Autodesk Fusion 360 part; units mm, degrees
sketch "Coupon chord" plane through (0, 0, 0) normal (0, 1, 0) x (1, 0, 0)
  line L0 (70, -76) -> (150, -76)
  line L1 (150, -76) -> (150, -90)
  line L2 (150, -90) -> (70, -90)
  line L3 (70, -90) -> (70, -76)
  dimension "d52" = 70
  dimension "d53" = 76
  dimension "d55" = 90
extrude "Coupon chord (1)" add sketch "Coupon chord" along normal mid plane 8
sketch "Saddle boss x=70" plane through (0, 0, 0) normal (0, 1, 0) x (1, 0, 0)
  circle A0 centre (70, -90) radius 22.7
  dimension "d58" = 70
  dimension "d59" = 90
  dimension "d60" = 45.4
extrude "Saddle boss x=70 (1)" add sketch "Saddle boss x=70" along normal mid plane 8
sketch "Saddle boss x=150" plane through (0, 0, 0) normal (0, 1, 0) x (1, 0, 0)
  circle A0 centre (150, -90) radius 22.7
  dimension "d64" = 90
  dimension "d65" = 45.4
extrude "Saddle boss x=150 (1)" add sketch "Saddle boss x=150" along normal mid plane 8
sketch "Rod pocket x=70" plane through (0, 0, 0) normal (0, 1, 0) x (1, 0, 0)
  circle A0 centre (70, -90) radius 17.1
  dimension "d68" = 70
  dimension "d69" = 90
  dimension "d70" = 34.2
extrude "Rod pocket x=70 (1)" cut sketch "Rod pocket x=70" along normal mid plane 18
sketch "Drop-in opening x=70" plane through (0, 0, 0) normal (0, 1, 0) x (1, 0, 0)
  line L0 (52.9, -90) -> (87.1, -90)
  line L1 (87.1, -90) -> (87.1, -117.7)
  line L2 (87.1, -117.7) -> (52.9, -117.7)
  line L3 (52.9, -117.7) -> (52.9, -90)
  dimension "d73" = 52.9
  dimension "d74" = 90
  dimension "d75" = 87.1
  dimension "d76" = 117.7
extrude "Drop-in opening x=70 (1)" cut sketch "Drop-in opening x=70" along normal mid plane 18
sketch "Rod pocket x=150" plane through (0, 0, 0) normal (0, 1, 0) x (1, 0, 0)
  circle A0 centre (150, -90) radius 17.1
  dimension "d80" = 90
  dimension "d81" = 34.2
extrude "Rod pocket x=150 (1)" cut sketch "Rod pocket x=150" along normal mid plane 18
sketch "Drop-in opening x=150" plane through (0, 0, 0) normal (0, 1, 0) x (1, 0, 0)
  line L0 (132.9, -90) -> (167.1, -90)
  line L1 (167.1, -90) -> (167.1, -117.7)
  line L2 (167.1, -117.7) -> (132.9, -117.7)
  line L3 (132.9, -117.7) -> (132.9, -90)
  dimension "d84" = 132.9
  dimension "d85" = 90
  dimension "d86" = 167.1
  dimension "d87" = 117.7
extrude "Drop-in opening x=150 (1)" cut sketch "Drop-in opening x=150" along normal mid plane 18
equation "couponWidth = 8.0 mm"
equation "plateHeight = 90.0 mm"
equation "rodOuterDiameter = 33.4 mm"
equation "saddleClearance = 0.8 mm"
equation "saddleWall = 6.0 mm"
equation "rearRodStandoff = 70.0 mm"
equation "rodSpacing = 80.0 mm"
equation "memberWidth = 14.0 mm"
equation "d52 = rearRodStandoff"
equation "d53 = plateHeight - memberWidth"
equation "d55 = plateHeight"
equation "d56 = couponWidth"
equation "d58 = rearRodStandoff"
equation "d59 = plateHeight"
equation "d60 = rodOuterDiameter + 2 * saddleWall"
equation "d61 = couponWidth"
equation "d64 = plateHeight"
equation "d65 = rodOuterDiameter + 2 * saddleWall"
equation "d66 = couponWidth"
equation "d68 = rearRodStandoff"
equation "d69 = plateHeight"
equation "d70 = rodOuterDiameter + saddleClearance"
equation "d71 = couponWidth + 10 mm"
equation "d73 = rearRodStandoff - ( rodOuterDiameter + saddleClearance ) / 2"
equation "d74 = plateHeight"
equation "d75 = rearRodStandoff + ( rodOuterDiameter + saddleClearance ) / 2"
equation "d76 = plateHeight + ( rodOuterDiameter + 2 * saddleWall ) / 2 + 5 mm"
equation "d77 = couponWidth + 10 mm"
equation "d80 = plateHeight"
equation "d81 = rodOuterDiameter + saddleClearance"
equation "d82 = couponWidth + 10 mm"
equation "d84 = ( rearRodStandoff + rodSpacing ) - ( rodOuterDiameter + saddleClearance ) / 2"
equation "d85 = plateHeight"
equation "d86 = ( rearRodStandoff + rodSpacing ) + ( rodOuterDiameter + saddleClearance ) / 2"
equation "d87 = plateHeight + ( rodOuterDiameter + 2 * saddleWall ) / 2 + 5 mm"
equation "d88 = couponWidth + 10 mm"
Model file for the job. Use its own axes, mm. A direction names the side the tool comes from. Give positions to 0.01 mm unless a question says otherwise; leave off trailing zeros. Loops run counter-clockwise (first coordinate to the right, second up) from the corner with the lowest first, then second, coordinate; pieces in that order, holes last.
1) Tool access for faces 4 (the flat face through (110, 0, 76)), 5 (the flat face through (132.9, 0, 98)), 6 (the cylindrical face through (164.86, 0.06, 72.84)): list every direction of +Z, -Z, +X, -X, +Y, -Y with a clear straight run to the whole face (end or side of a thin tool).
2) Pull direction X, two halves, no side cores. Call faces 1 (the flat face through (110, -4, 79)), 2 (the flat face through (52.9, 0, 98)), 3 (the cylindrical face through (55.925, 0.056, 72.19)): +X half, -X half, draft (parallel to the pull), parting line (faces both ways), or undercut.
3) Saw through at D-D (x = 150). Write the cut outline in (y, z).
4) Saw through at B-B (z = 83). Write the cut outline in (x, y).
5) Saw through at C-C (z = 71). Write the cut outline in (x, y).
6) Flat gauge pins, fed straight in: pin 1 Ø4 at (x, y) = (132, -1.5) entering from -Z; pin 2 Ø2 at (y, z) = (0.5, 72) entering from -X; pin 3 Ø3 at (x, y) = (100.5, 3) entering from -Z. Where does each tip first touch, or does it go through?
7) Wall check: line 1 (X direction, y = 1.5, z = 93); line 2 (X direction, y = 3, z = 94); line 3 (X direction, y = 0, z = 78.5). Give the ranges that are in metal, low to high.
8) Saw through at A-A (y = -2.5). Write the cut outline in (x, z), plus the area to 3 significant figures.
Answer block:
1. face 4: -Z, +Y, -Y
1. face 5: +Z, +Y, -Y
1. face 6: +Y, -Y
2. face 1: draft
2. face 2: undercut
2. face 3: undercut
3. outline: (-4, 67.3) - (4, 67.3) - (4, 72.9) - (-4, 72.9) - close
4. outline: (48.41, -4) - (54.4, -4) - (54.4, 4) - (48.41, 4) - close; (85.6, -4) - (134.4, -4) - (134.4, 4) - (85.6, 4) - close; (165.6, -4) - (171.59, -4) - (171.59, 4) - (165.6, 4) - close
5. outline: (57.58, -4) - (82.42, -4) - (82.42, 4) - (57.58, 4) - close; (137.58, -4) - (162.42, -4) - (162.42, 4) - (137.58, 4) - close
6. pin 1: stops at z = 73.9
6. pin 2: stops at x = 54.96
6. pin 3: stops at z = 76
7. line 1: x = 47.5 to 52.9, 87.1 to 92.5, 127.5 to 132.9, 167.1 to 172.5
7. line 2: x = 47.66 to 52.9, 87.1 to 92.34, 127.66 to 132.9, 167.1 to 172.34
7. line 3: x = 50.43 to 57.34, 82.66 to 137.34, 162.66 to 169.57
8. outline: (52.9, 90) - (52.9, 104.93) arc R22.7 ccw (long way) to (87.87, 76) - (132.13, 76) arc R22.7 ccw (long way) to (167.1, 104.93) - (167.1, 90) arc R17.1 cw to (132.9, 90) - (132.9, 104.93) arc R22.7 ccw to (127.3, 90) - (92.7, 90) arc R22.7 ccw to (87.1, 104.93) - (87.1, 90) arc R17.1 cw to start
8. area: 1,460 mm2
